Here's how the part is built. I have some questions about the finished solid (model axes, mm). Give positions to 0.01 mm unless a question says otherwise; leave off trailing zeros. Loops run counter-clockwise (first coordinate to the right, second up) from the corner with the lowest first, then second, coordinate; pieces in that order, holes last.
Q1. I need wall thicknesses on line 1 (Z direction, x = -11.5, y = 3.95); line 2 (X direction, y = 4.7, z = 8); line 3 (X direction, y = 1.25, z = 12). Which ranges of each line are inside material? Lowest first, please.
Q2. If we section it at D-D (y = 3.3): Give the number of separate pieces and of enclosed holes in the cut face, plus the area to 3 significant figures.
Q3. Will these pins go through, and if not, where does the flat tip stop? P1, Ø1, axis at y = 1, z = -38, coming from the -X side; P2, Ø2, axis at y = 1, z = -33.5, coming from the -X side; P3, Ø7.5, axis at x = -67, z = -13, coming from the -Y side; P4, Ø3, axis at x = 70.5, y = 1, coming from the -Z side.
Q4. If we section it at B-B (z = -34.5): Please give me the cut outline in (x, y).
Q5. If we section it at C-C (z = -1): Please give me the cut outline in (x, y), plus the area to 3 significant figures.
Q6. If we section it at A-A (x = -67): Please give me the cut outline in (y, z).
Autodesk Inventor part; units mm, degrees
ref_plane "YZ Plane" through (0, 0, 0) normal (1, 0, 0) x (0, 1, 0)
ref_plane "XZ Plane" through (0, 0, 0) normal (0, 1, 0) x (-1, 0, 0)
ref_plane "XY Plane" through (0, 0, 0) normal (0, 0, 1) x (1, 0, 0)
sketch "Sketch1" plane through (0, 0, 0) normal (0, 1, 0) x (-1, 0, 0)
  line L0 (-115, -52.5) -> (115, -52.5)
  line L1 (115, -52.5) -> (115, 52.5)
  line L2 (115, 52.5) -> (-115, 52.5)
  line L3 (-115, 52.5) -> (-115, -52.5)
  line L4 (-115, -52.5) -> (115, 52.5) construction
  line L5 (115, -52.5) -> (-115, 52.5) construction
  line L6 (-108, 13) -> (-67, 13) construction
  line L7 (-67, 13) -> (-67, -13) construction
  line L8 (-67, -13) -> (-108, -13) construction
  line L9 (-108, -13) -> (-108, 13) construction
  line L10 (-108, 13) -> (-67, -13) construction
  line L11 (-67, 13) -> (-108, -13) construction
  line L12 (67, 13) -> (108, 13) construction
  line L13 (108, 13) -> (108, -13) construction
  line L14 (108, -13) -> (67, -13) construction
  line L15 (67, -13) -> (67, 13) construction
  line L16 (67, 13) -> (108, -13) construction
  line L17 (108, 13) -> (67, -13) construction
  circle A0 centre (-67, 13) radius 2.4
  circle A1 centre (-67, -13) radius 2.4
  circle A2 centre (-108, -13) radius 2.4
  circle A3 centre (-108, 13) radius 2.4
  circle A4 centre (67, 13) radius 2.4
  circle A5 centre (108, 13) radius 2.4
  circle A6 centre (108, -13) radius 2.4
  circle A7 centre (67, -13) radius 2.4
  line L18 (-37.5, -40) -> (37.5, -40)
  line L19 (37.5, -40) -> (37.5, 40)
  line L20 (37.5, 40) -> (-37.5, 40)
  line L21 (-37.5, 40) -> (-37.5, -40)
  line L22 (-37.5, -40) -> (37.5, 40) construction
  line L23 (37.5, -40) -> (-37.5, 40) construction
  point P0 (0, 0)
  point P1 (-87.5, 0)
  point P2 (87.5, 0)
  dimension "d0" = 105
  dimension "d3" = 26
  dimension "d4" = 41
  dimension "d5" = 175
  dimension "d6" = 87.5
  dimension "d7" = 230
  dimension "d8" = 4.8
  dimension "d9" = 80
  dimension "d10" = 75
extrude "Extrusion1" add sketch "Sketch1" along normal blind 5.588
sketch "Sketch2" plane through (0, 0, 0) normal (0, -1, 0) x (1, 0, 0)
  line L0 (115, -52.5) -> (-115, -52.5)
  line L1 (115, 52.5) -> (115, -52.5)
  line L2 (-115, 52.5) -> (115, 52.5)
  line L3 (-115, -52.5) -> (-115, 52.5)
  line L4 (-115, 52.5) -> (-115, 22.5)
  line L5 (-115, 22.5) -> (-55, 52.5)
  line L6 (-55, 52.5) -> (-115, 52.5)
  line L7 (-115, -22.5) -> (-115, -52.5)
  line L8 (-115, -52.5) -> (-55, -52.5)
  line L9 (-115, -22.5) -> (-55, -52.5)
  line L10 (55, 52.5) -> (115, 22.5)
  line L11 (115, 22.5) -> (115, 52.5)
  line L12 (115, 52.5) -> (55, 52.5)
  line L13 (115, -22.5) -> (115, -52.5)
  line L14 (115, -52.5) -> (55, -52.5)
  line L15 (55, -52.5) -> (115, -22.5)
  point P0 (0, 0)
  dimension "d13" = 60
  dimension "d14" = 30
extrude "Extrusion2" cut sketch "Sketch2" against normal blind 10 contours L0 L15 L1 | L0 L3 L9 | L10 L2 L1 | L3 L2 L5
fillet "Fillet1" radius 25 8 edges at (-55, 2.794, -52.5) (-115, 2.794, -22.5) (55, 2.794, -52.5) (115, 2.794, -22.5) (115, 2.794, 22.5) (55, 2.794, 52.5) (-55, 2.794, 52.5) (-115, 2.794, 22.5)
sketch "Sketch4" plane through (0, 0, 0) normal (0, -1, 0) x (1, 0, 0)
  line L0 (55, -25) -> (-55, -25) construction
  line L1 (-55, -25) -> (-55, 25) construction
  line L2 (-55, 25) -> (55, 25) construction
  line L3 (55, 25) -> (55, -25) construction
  line L4 (55, -25) -> (-55, 25) construction
  line L5 (-55, -25) -> (55, 25) construction
  circle A0 centre (-55, 25) radius 2
  circle A1 centre (-55, -25) radius 2
  circle A2 centre (55, -25) radius 2
  circle A3 centre (55, 25) radius 2
  point P0 (0, 0)
  dimension "d18" = 4
  dimension "d20" = 50
  dimension "d23" = 110
extrude "Extrusion3" cut sketch "Sketch4" against normal blind 10
fillet "Fillet2" radius 8 4 edges at (-37.5, 2.794, 40) (37.5, 2.794, 40) (-37.5, 2.794, -40) (37.5, 2.794, -40)
properties part number "VatPlate"
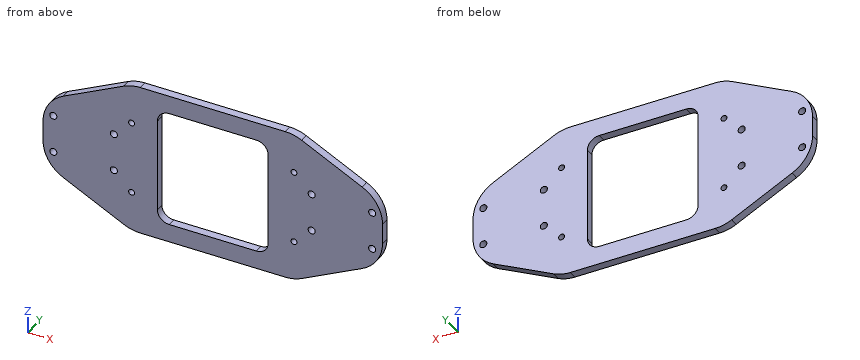
Check sheet entries:
1. line 1: z = -52.5 to -40, 40 to 52.5
1. line 2: x = -114.98 to -37.5, 37.5 to 114.98
1. line 3: x = -114.5 to -110.18, -105.82 to -69.18, -64.82 to -37.5, 37.5 to 64.82, 69.18 to 105.82, 110.18 to 114.5
2. separate pieces: 1
2. enclosed holes: 13
2. area: 14,200 mm2
3. P1: stops at x = -85
3. P2: stops at x = -95
3. P3: stops at y = 0
3. P4: stops at z = -45.5
4. outline: (-91, 0) - (-37.1, 0) - (-37.1, 5.59) - (-91, 5.59) - close; (37.1, 0) - (91, 0) - (91, 5.59) - (37.1, 5.59) - close
5. outline: (-115, 0) - (-37.5, 0) - (-37.5, 5.59) - (-115, 5.59) - close; (37.5, 0) - (115, 0) - (115, 5.59) - (37.5, 5.59) - close
5. area: 866 mm2
6. outline: (0, -46.5) - (5.59, -46.5) - (5.59, -15.4) - (0, -15.4) - close; (0, -10.6) - (5.59, -10.6) - (5.59, 10.6) - (0, 10.6) - close; (0, 15.4) - (5.59, 15.4) - (5.59, 46.5) - (0, 46.5) - close
